Print and shaded views of the part. All mm, measured from the part's lowest x, y and z. Round coordinates to 2 decimals unless told otherwise and drop trailing zeros. Order: outer loops, then holes, each group sorted by start corner. A loop starts at its lowest first (then second) coordinate and runs counter-clockwise, first axis right, second up. Notation, with made-up numbers: (-28.5, -7.5) -> (9.5, -7.5) arc R25 ccw to (9.5, 23.5) -> close; hole circle Ø5 at (-40, -8.5). An arc over 180 degrees is marked (long way). Answer as CSV lines item,"result".
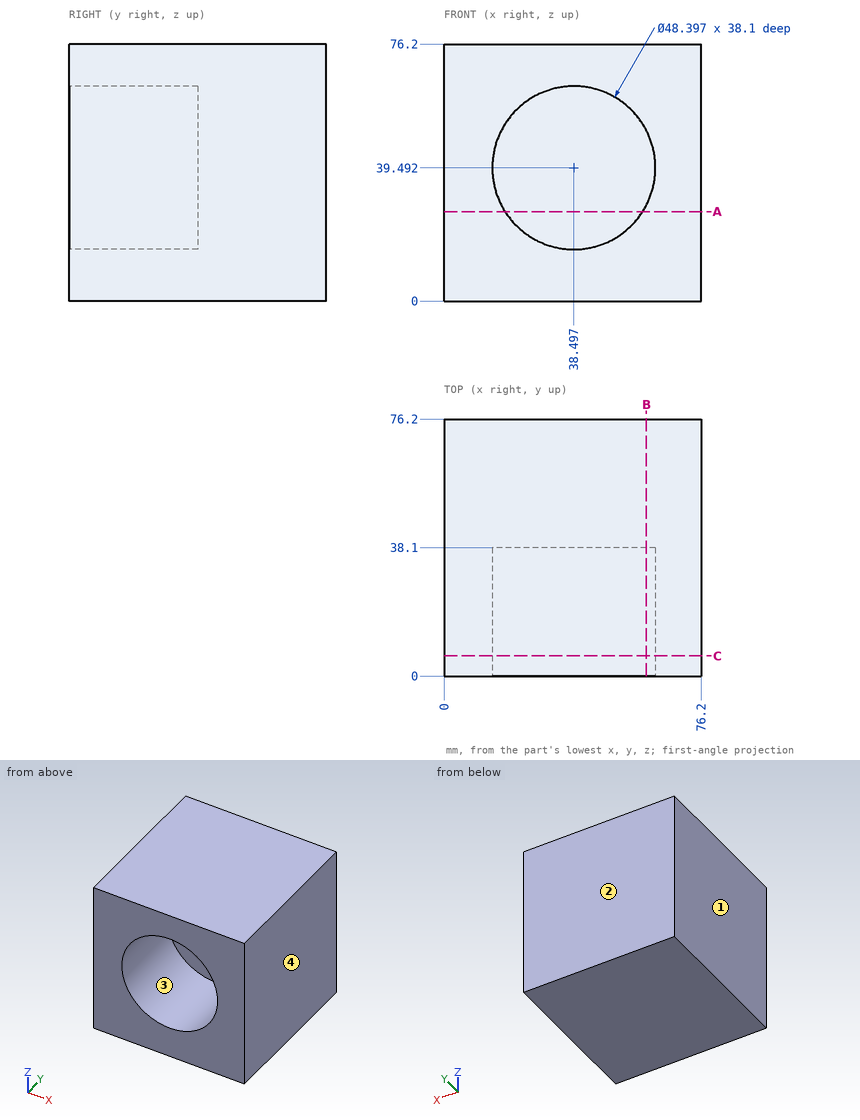
Q1. Saw through at B-B (x = 60). Write the cut outline in (y, z), plus the area to 3 significant figures.
Checks:
outline,"(0, 0) -> (76.2, 0) -> (76.2, 76.2) -> (0, 76.2) -> (0, 50.59) -> (38.1, 50.59) -> (38.1, 28.39) -> (0, 28.39) -> close"
area,"4,960 mm²"
Q2. Wall check: L1, parallel to Y at x = 25, z = 21; L2, parallel to X at y = 15.5, z = 32.5; L3, parallel to Z at x = 34, y = 7.5 (1 decimal). Give the ranges that are in metal, low to high. Write a range as [from, to].
Checks:
L1,"[38.1, 76.2]"
L2,"[0, 15.33], [61.66, 76.2]"
L3,"[0, 15.7], [63.3, 76.2]"
Q3. Mould opens along X. For the marked faces 1, 2, 3 and 4 say: +X half, -X half, draft (parallel to the pull), parting line (faces both ways), or undercut.
Checks:
face 1,"-X half"
face 2,"draft"
face 3,"undercut"
face 4,"+X half"
Q4. Saw through at C-C (y = 6). Write the cut outline in (x, z), plus the area to 3 significant figures.
Checks:
outline,"(0, 0) -> (76.2, 0) -> (76.2, 76.2) -> (0, 76.2) -> close; hole circle Ø48.4 at (38.5, 39.49)"
area,"3,970 mm²"
Q5. Saw through at A-A (z = 26.5). Write the cut outline in (x, y), plus the area to 3 significant figures.
Checks:
outline,"(0, 0) -> (18.08, 0) -> (18.08, 38.1) -> (58.91, 38.1) -> (58.91, 0) -> (76.2, 0) -> (76.2, 76.2) -> (0, 76.2) -> close"
area,"4,250 mm²"
Q6. Flat gauge pins, fed straight in: pin 1 (1 mm diameter, centred on y = 28, z = 35, fed in from -X); pin 2 (1.5 mm diameter, centred on x = 24.5, z = 21, fed in from -Y). Where does each tip first touch, or does it go through?
Checks:
pin 1,"x = 0"
pin 2,"y = 38.1"
